Check sheet for the modelled part. Datum: model origin and axes. Units: mm. A direction names the side the tool comes from. Give positions to 0.01 mm unless a question says otherwise; leave off trailing zeros. Order: outer loops, then holes, each group sorted by start corner. A loop starts at its lowest first (then second) coordinate and runs counter-clockwise, first axis right, second up.
Item 1: Sectioned sample at A-A on x = -9.5. Record the boundary of the cut face in (y, z) (3 decimals), and give its area (3 significant figures).
Item 2: Release check for a two-part mould opening along X. For faces 1 (the flat face through (22, -18.146, 12)), 2 (the flat face through (-14.844, 23, 10)), 3 (the flat face through (18.146, 22, 8)), 4 (the flat face through (-15.113, -22, 8)) record: released by +X, released by -X, zero draft, split by the parting line, or undercut.
Item 3: Material ranges on line 1 along Y through (x, z) = (20.5, 12.5); line 2 along Z through (x, y) = (14, 12) (3 decimals); line 3 along Y through (x, z) = (19, 7.25), recorded low to high.
Item 4: Gauge pin test, flat ends, axial feed: P1, Ø5.5, axis at y = -22, z = 8, coming from the -X side (3 decimals); P2, Ø1.7, axis at x = 16.5, y = -22, coming from the -Z side; P3, Ø4, axis at x = 21.5, z = 7, coming from the -Y side; P4, Ø7, axis at x = 16.002, y = -16.002, coming from the +Z side. Record the tip position at first contact, or that the pin passes through.
Item 5: Access from +Z, -Z, +X, -X, +Y, -Y to the whole of each face (thin tool, end or side, straight path). Record for faces 5 (the flat face through (22, 17, 18.628)), 6 (the cylindrical face through (-16.79, -22.87, 16.24)), 7 (the flat face through (-17, -22, 0.849)).
Item 6: Sectioned sample at C-C on x = 17. Count the separate pieces of the cut face and the enclosed holes in it, and give its area (3 significant figures).
from build123d import *

# Parameters (mm, degrees)
F0_R      = 2.159
F1_DEPTH  = 21.082
F2_W      = 26.162
F2_H      = 17.272
F4_DEPTH  = 38.355
F3_W      = 26.162
F3_H      = 17.272
F5_DEPTH  = 38.355
F2_W_2    = 0.635
F2_H_2    = 17.7696704889
F6_DEPTH  = 5.08
F3_W_2    = 0.635
F3_H_2    = 17.78
F7_DEPTH  = 5.08
F9_W      = 3.302
F9_H      = 17.9293047404
F10_DEPTH = 5.08
F8_W      = 0.635
F8_H      = 17.9293047404
F11_DEPTH = 5.08
F12_R     = 1.2446
F12_R_2   = 1.651
F13_DEPTH = 11.43
F14_R     = 1.2446
F14_R_2   = 1.651
F15_DEPTH = 11.43
F16_R     = 1.524
F16_R_2   = 1.2446
F17_DEPTH = 11.43
F19_R     = 1.2446
F19_R_2   = 1.651
F20_DEPTH = 11.43
F21_W     = 25.399999693
F21_H     = 25.399999693
F22_DEPTH = 21.083
F23_DEPTH = 2.667
F24_DEPTH = 2.667
F25_DEPTH = 2.667
F26_DEPTH = 2.667
F27_DEPTH = 2.667
F28_DEPTH = 2.667
F29_R     = 1.0414
F30_DEPTH = 11.43
F32_R     = 1.0414
F33_DEPTH = 11.43
F34_R     = 1.0414
F35_DEPTH = 11.43
F36_R     = 1.0414
F37_DEPTH = 11.43


with BuildPart() as f1:
    # F0 (on Top) → F1 (new body)
    with BuildSketch(Plane.XY):
        Polygon((17.906382707, 19.177), (-17.907, 19.177), (-19.177, 19.177), (-19.177, 17.907), (-19.177, -17.907), (-19.177, -19.177), (-17.9054846503, -19.177), (17.907, -19.177), (19.177, -19.177), (19.177, -17.907), (19.177, 17.907), (19.177, 19.177), (17.907, 19.177), align=None)
        with Locations((-16.002, -16.002)):
            Circle(F0_R, mode=Mode.SUBTRACT)
        with Locations((16.002, -16.002)):
            Circle(F0_R, mode=Mode.SUBTRACT)
        with Locations((-16.002, 16.002)):
            Circle(F0_R, mode=Mode.SUBTRACT)
        with Locations((16.002, 16.002)):
            Circle(F0_R, mode=Mode.SUBTRACT)
    extrude(amount=F1_DEPTH)

    # F2 (on face) → F4 (cut, through all)
    with BuildSketch(Plane.XZ.offset(19.177)):
        with Locations((0.3429, 10.541)):
            Rectangle(F2_W, F2_H)
    extrude(amount=-F4_DEPTH, mode=Mode.SUBTRACT)

    # F3 (on face) → F5 (cut, through all)
    with BuildSketch(Plane.YZ.offset(19.177)):
        with Locations((0.3429, 10.541)):
            Rectangle(F3_W, F3_H)
    extrude(amount=-F5_DEPTH, mode=Mode.SUBTRACT)

    # F2 (on face) → F6 (join)
    with BuildSketch(Plane.XZ.offset(19.177)):
        with Locations((18.0975, 9.7333647556)):
            Rectangle(F2_W_2, F2_H_2)
        with Locations((-18.0975, 9.7333647556)):
            Rectangle(F2_W_2, F2_H_2)
    extrude(amount=F6_DEPTH)

    # F3 (on face) → F7 (join)
    with BuildSketch(Plane.YZ.offset(19.177)):
        with Locations((-17.828373853, 9.73836)):
            Rectangle(F3_W_2, F3_H_2)
        with Locations((17.828373853, 9.73836)):
            Rectangle(F3_W_2, F3_H_2)
    extrude(amount=F7_DEPTH)

    # F9 (on face) → F10 (join)
    with BuildSketch(Plane(origin=(0, 19.177, 0), x_dir=(-1, 0, 0), z_dir=(0, 1, 0))):
        with Locations((-16.49476, 10.2123476298)):
            Rectangle(F9_W, F9_H)
        with Locations((16.49476, 10.2123476298)):
            Rectangle(F9_W, F9_H)
    extrude(amount=F10_DEPTH)

    # F8 (on face) → F11 (join)
    with BuildSketch(Plane(origin=(-19.177, 0, 0), x_dir=(0, -1, 0), z_dir=(-1, 0, 0))):
        with Locations((-18.2245, 10.2123476298)):
            Rectangle(F8_W, F8_H)
        with Locations((18.2245, 10.2123476298)):
            Rectangle(F8_W, F8_H)
    extrude(amount=F11_DEPTH)

    # F12 (on face) → F13 (cut)
    with BuildSketch(Plane(origin=(0, 18.542, 0), x_dir=(-1, 0, 0), z_dir=(0, 1, 0))):
        with Locations((21.717, 3.1526952596)):
            Circle(F12_R)
        with Locations((21.717, 6.3276952596)):
            Circle(F12_R_2)
        with Locations((21.717, 9.5026952596)):
            Circle(F12_R)
    extrude(amount=-F13_DEPTH, mode=Mode.SUBTRACT)

    # F14 (on face) → F15 (cut)
    with BuildSketch(Plane.YZ.offset(18.14576)):
        with Locations((21.717, 10.8458)):
            Circle(F14_R)
        with Locations((21.717, 14.097)):
            Circle(F14_R_2)
        with Locations((21.717, 17.272)):
            Circle(F14_R)
    extrude(amount=-F15_DEPTH, mode=Mode.SUBTRACT)

    # F16 (on face) → F17 (cut)
    with BuildSketch(Plane(origin=(-18.415, 0, 0), x_dir=(0, -1, 0), z_dir=(-1, 0, 0))):
        with Locations((21.717, 13.5382)):
            Circle(F16_R)
        with Locations((21.717, 10.3632)):
            Circle(F16_R_2)
        with Locations((21.717, 16.7132)):
            Circle(F16_R_2)
    extrude(amount=-F17_DEPTH, mode=Mode.SUBTRACT)

    # F19 (on face) → F20 (cut)
    with BuildSketch(Plane.XZ.offset(18.145873853)):
        with Locations((21.717, 2.75336)):
            Circle(F19_R)
        with Locations((21.717, 5.92836)):
            Circle(F19_R_2)
        with Locations((21.717, 9.10336)):
            Circle(F19_R)
    extrude(amount=-F20_DEPTH, mode=Mode.SUBTRACT)

    # F21 (on face) → F22 (cut, through all)
    with BuildSketch(Plane.XY.offset(21.082)):
        Rectangle(F21_W, F21_H)
    extrude(amount=-F22_DEPTH, mode=Mode.SUBTRACT)

    # F23 (add): a face of the model
    f23_faces = [f1.faces().sort_by_distance(p)[0] for p in [
        (-21.717, 17.907, 11.1888492438),
    ]]
    extrude(f23_faces, amount=F23_DEPTH)

    # F24 (add): a face of the model
    f24_faces = [f1.faces().sort_by_distance(p)[0] for p in [
        (-21.717, -17.907, 10.2123476298),
    ]]
    extrude(f24_faces, amount=F24_DEPTH)

    # F25 (add): a face of the model
    f25_faces = [f1.faces().sort_by_distance(p)[0] for p in [
        (17.78, -21.717, 9.7333647556),
    ]]
    extrude(f25_faces, amount=F25_DEPTH)

    # F26 (add): a face of the model
    f26_faces = [f1.faces().sort_by_distance(p)[0] for p in [
        (-17.78, -21.717, 8.8486881726),
    ]]
    extrude(f26_faces, amount=F26_DEPTH)

    # F27 (add): a face of the model
    f27_faces = [f1.faces().sort_by_distance(p)[0] for p in [
        (21.717, -17.510873853, 10.7061813162),
    ]]
    extrude(f27_faces, amount=F27_DEPTH)

    # F28 (add): a face of the model
    f28_faces = [f1.faces().sort_by_distance(p)[0] for p in [
        (21.717, 17.510873853, 9.73836),
    ]]
    extrude(f28_faces, amount=F28_DEPTH)

    # F29 (on face) → F30 (cut)
    with BuildSketch(Plane(origin=(0, 18.145873853, 0), x_dir=(-1, 0, 0), z_dir=(0, 1, 0))):
        with Locations((-21.717, 5.9341536835)):
            Circle(F29_R)
        with Locations((-21.717, 9.10336)):
            Circle(F29_R)
        with Locations((-21.717, 2.7551189996)):
            Circle(F29_R)
    extrude(amount=-F30_DEPTH, mode=Mode.SUBTRACT)

    # F32 (on face) → F33 (cut)
    with BuildSketch(Plane(origin=(-18.14576, 0, 0), x_dir=(0, -1, 0), z_dir=(-1, 0, 0))):
        with Locations((-21.717, 17.272)):
            Circle(F32_R)
        with Locations((-21.717, 14.097)):
            Circle(F32_R)
        with Locations((-21.717, 10.922)):
            Circle(F32_R)
    extrude(amount=-F33_DEPTH, mode=Mode.SUBTRACT)

    # F34 (on face) → F35 (cut)
    with BuildSketch(Plane.XZ.offset(18.542)):
        with Locations((-21.717, 9.5026952596)):
            Circle(F34_R)
        with Locations((-21.717, 6.3276952596)):
            Circle(F34_R)
        with Locations((-21.717, 3.1526952596)):
            Circle(F34_R)
    extrude(amount=-F35_DEPTH, mode=Mode.SUBTRACT)

    # F36 (on face) → F37 (cut)
    with BuildSketch(Plane.YZ.offset(18.415)):
        with Locations((-21.717, 16.7132)):
            Circle(F36_R)
        with Locations((-21.717, 13.5382)):
            Circle(F36_R)
        with Locations((-21.717, 10.3632)):
            Circle(F36_R)
    extrude(amount=-F37_DEPTH, mode=Mode.SUBTRACT)


solid = f1.part
Report:
1. outline: (-19.177, 0) - (-12.7, 0) - (-12.7, 1.905) - (-19.177, 1.905) - close; (-19.177, 19.177) - (-12.7, 19.177) - (-12.7, 21.082) - (-19.177, 21.082) - close; (12.7, 0) - (19.177, 0) - (19.177, 1.905) - (12.7, 1.905) - close; (12.7, 19.177) - (19.177, 19.177) - (19.177, 21.082) - (12.7, 21.082) - close
1. area: 49.4 mm2
2. face 1: zero draft
2. face 2: undercut
2. face 3: released by +X
2. face 4: undercut
3. line 1: y = -18.15 to -14.84, 14.84 to 18.15
3. line 2: z = 0 to 1.905, 19.177 to 21.082
3. line 3: y = -19.18 to -12.74, 13.42 to 19.18
4. P1: stops at x = -18.415
4. P2: stops at z = 0.85
4. P3: stops at y = -18.15
4. P4: stops at z = 21.08
5. face 5: +Z, +X, +Y, -Y
5. face 6: -X
5. face 7: -Z, +X, -X, -Y
6. separate pieces: 3
6. enclosed holes: 7
6. area: 348 mm2
